from build123d import *

# Parameters (mm, degrees)
F1_DEPTH = 10.05
F2_R     = 7.5
F3_DEPTH = 25


with BuildPart() as f1:
    # F0 (on Front) → F1 (new body, symmetric)
    with BuildSketch(Plane.XZ):
        with BuildLine():
            ThreePointArc((-34.677416, 6.798443), (-30.284018, -3.808158), (-19.677416, -8.201557))
            Line((-19.677416, -8.201557), (50.862584, -8.201557))
            ThreePointArc((50.862584, -8.201557), (61.469185, -3.808158), (65.862584, 6.798443))
            Line((65.862584, 6.798443), (65.862584, 42.354545))
            Line((65.862584, 42.354545), (45.862584, 42.354545))
            Line((45.862584, 42.354545), (45.862584, 11.901609))
            Line((45.862584, 11.901609), (-12.677416, 11.901609))
            Line((-12.677416, 11.901609), (-12.677416, 42.704577))
            Line((-12.677416, 42.704577), (-34.677416, 42.704577))
            Line((-34.677416, 42.704577), (-34.677416, 6.798443))
        make_face()
    extrude(amount=F1_DEPTH, both=True)

    # F2 (on face) → F3 (cut)
    with BuildSketch(Plane(origin=(-34.677416, 0, 0), x_dir=(0, -1, 0), z_dir=(-1, 0, 0))):
        with Locations((0, 31.453513)):
            Circle(F2_R)
    extrude(amount=-F3_DEPTH, mode=Mode.SUBTRACT)


solid = f1.part
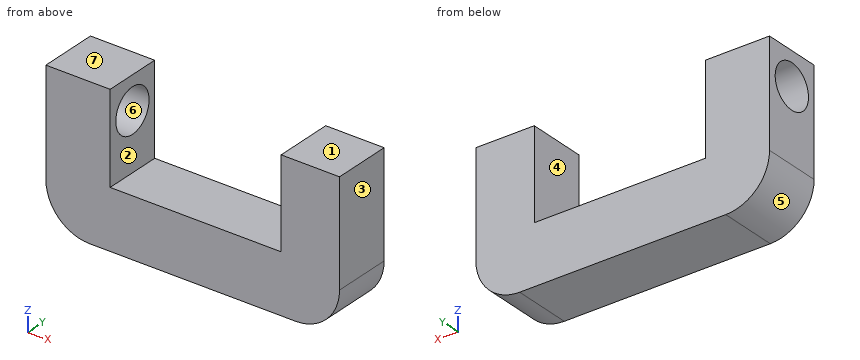
CAD build for the part. Positions are in the model's coordinates, mm. Face numbers are marked on the shaded views. A direction names the side the tool comes from. Coordinates: 2 decimals unless noted, no trailing zeros. Order: outer loops, then holes, each group sorted by start corner. A loop starts at its lowest first (then second) coordinate and runs counter-clockwise, first axis right, second up.
Item 1: Two-plate mould, pull along Z, no slides. Class the marked faces 4, 5, 6 and 7: +Z half, -Z half, draft (parallel to the pull), parting line (faces both ways), or undercut.
Check sheet entries:
face 4: draft
face 5: -Z half
face 6: undercut
face 7: +Z half
Item 2: Drill centre lines: L1, parallel to X at y = 0.5, z = 39; L2, parallel to X at y = 8.25, z = 6.5; L3, parallel to Z at x = -23, y = 0. Where is each one in solid material? Low to high.
Check sheet entries:
L1: x = -34.68 to -12.68, 45.86 to 65.86
L2: x = -34.67 to 65.86
L3: z = -7.83 to 23.95, 38.95 to 42.7
Item 3: Band-saw the part on B-B on z = 34. List the corners of the cut face in (x, y).
Check sheet entries:
outline: (-34.68, -10.05) - (-12.68, -10.05) - (-12.68, -7.05) - (-34.68, -7.05) - close; (-34.68, 7.05) - (-12.68, 7.05) - (-12.68, 10.05) - (-34.68, 10.05) - close; (45.86, -10.05) - (65.86, -10.05) - (65.86, 10.05) - (45.86, 10.05) - close
Item 4: Pin check, flat tips, straight feed: pin 1 Ø10 at (x, y) = (55.5, -0.5) entering from +Z; pin 2 Ø8 at (x, y) = (21, -5.5) entering from +Z; pin 3 Ø3 at (y, z) = (4, -1.5) entering from +X. Stop position of each tip, or through.
Check sheet entries:
pin 1: stops at z = 42.35
pin 2: stops at z = 11.9
pin 3: stops at x = 64.23
Item 5: Band-saw the part on C-C on x = 21. List the corners of the cut face in (y, z).
Check sheet entries:
outline: (-10.05, -8.2) - (10.05, -8.2) - (10.05, 11.9) - (-10.05, 11.9) - close
Item 6: Band-saw the part on A-A on y = 0. List the corners of the cut face in (x, z), plus the area to 3 significant figures.
Check sheet entries:
outline: (-34.68, 6.8) arc R15 ccw to (-19.68, -8.2) - (50.86, -8.2) arc R15 ccw to (65.86, 6.8) - (65.86, 42.35) - (45.86, 42.35) - (45.86, 11.9) - (-12.68, 11.9) - (-12.68, 23.95) - (-34.68, 23.95) - close; (-34.68, 38.95) - (-12.68, 38.95) - (-12.68, 42.7) - (-34.68, 42.7) - close
area: 2,880 mm2
Item 7: 3-axis set-ups, long thin cutter, end or side, ignore diameter. For the marked faces 1, 2 and 3: which of +Z, -Z, +X, -X, +Y, -Y reach the whole face in a straight line?
Check sheet entries:
face 1: +Z, +X, +Y, -Y
face 2: +Z, +Y, -Y
face 3: +Z, -Z, +X, +Y, -Y
Item 8: Band-saw the part on D-D on y = -5.5. List the corners of the cut face in (x, z), plus the area to 3 significant figures.
Check sheet entries:
outline: (-34.68, 6.8) arc R15 ccw to (-19.68, -8.2) - (50.86, -8.2) arc R15 ccw to (65.86, 6.8) - (65.86, 42.35) - (45.86, 42.35) - (45.86, 11.9) - (-12.68, 11.9) - (-12.68, 26.35) - (-34.68, 26.35) - close; (-34.68, 36.55) - (-12.68, 36.55) - (-12.68, 42.7) - (-34.68, 42.7) - close
area: 2,990 mm2
